The listing builds one solid part. Answer for the finished solid, in the listing's coordinates (mm). A direction names the side the tool comes from. Give positions to 0.01 mm unless a question says otherwise; leave off trailing zeros. Order: outer loops, then holes, each group sorted by start corner. A loop starts at its lowest first (then second) coordinate and runs counter-clockwise, first axis right, second up. Notation, with made-up numbers: (84.25, 22) - (118.25, 22) arc R13 cw to (118.25, 31) - close; hole circle Ø10 at (24, 9). An arc over 180 degrees is marked (long way). Answer as a JSON object with one key per item and string values. Group by question number.
Q1. The mould has two halves that part along Y. Classify faces 1 (the face through (12, 12, -2)), 2 (the face through (12, -1, 1)), 3 (the face through (24, 12, 1)), 4 (the face through (12, 25.5, 1)): released by +Y, released by -Y, zero draft, split by the parting line, or undercut.
Q2. Consider line 1 (Y direction, x = 9, z = 1.9); line 2 (X direction, y = 10.75, z = 1.45); line 3 (Z direction, x = 17, y = 14.5). Determine where each line is inside the solid, lowest interval first.
Q3. A cutting plane is placed at A-A, the plane z = 2.65. Give the vertices of the cut face in (x, y).
Q4. Given pin 1 (7 mm diameter, centred on x = 16, y = 13, fed in from +Z), flat-ended and moving along its own axis, determine where the tip first touches the part or whether it passes through.
Q5. A cutting plane is placed at B-B, the plane x = 2.5. Give the vertices of the cut face in (y, z).
Q6. A cutting plane is placed at C-C, the plane y = 20.75. Give the vertices of the cut face in (x, z).
Q7. For faces 5 (the face through (-0.6, 12.3, 3)), 6 (the face through (12, 12, 0)), determine the directions among +Z, -Z, +X, -X, +Y, -Y from which every point of the face is accessible in a straight line to the end or side of a thin tool.
from build123d import *

# Parameters (mm, degrees)
SKETCH_1_W      = 26
SKETCH_1_H      = 26.5
SKETCH_1_W_2    = 24
SKETCH_1_H_2    = 24.5
EXTRUDE_1_DEPTH = 3
SKETCH_2_W      = 26
SKETCH_2_H      = 26.5
EXTRUDE_2_DEPTH = 2


with BuildPart() as part:
    # 草图1 → 凸台-拉伸1 (new body)
    with BuildSketch(Plane.XY):
        with Locations((12, 12.25)):
            Rectangle(SKETCH_1_W, SKETCH_1_H)
        with Locations((12, 12.25)):
            Rectangle(SKETCH_1_W_2, SKETCH_1_H_2, mode=Mode.SUBTRACT)
    extrude(amount=EXTRUDE_1_DEPTH)

    # 草图2 → 凸台-拉伸2 (add)
    with BuildSketch(Plane(origin=(0, 0, 0), x_dir=(-1, 0, 0), z_dir=(0, 0, -1))):
        with Locations((-12, 12.25)):
            Rectangle(SKETCH_2_W, SKETCH_2_H)
    extrude(amount=EXTRUDE_2_DEPTH)


solid = part.part
Reply:
{
 "1": {"face 1": "zero draft", "face 2": "released by -Y", "face 3": "undercut", "face 4": "released by +Y"},
 "2": {"line 1": "y = -1 to 0, 24.5 to 25.5", "line 2": "x = -1 to 0, 24 to 25", "line 3": "z = -2 to 0"},
 "3": {"outline": "(-1, -1) - (25, -1) - (25, 25.5) - (-1, 25.5) - close; hole (0, 0) - (24, 0) - (24, 24.5) - (0, 24.5) - close"},
 "4": {"pin 1": "stops at z = 0"},
 "5": {"outline": "(-1, -2) - (25.5, -2) - (25.5, 3) - (24.5, 3) - (24.5, 0) - (0, 0) - (0, 3) - (-1, 3) - close"},
 "6": {"outline": "(-1, -2) - (25, -2) - (25, 3) - (24, 3) - (24, 0) - (0, 0) - (0, 3) - (-1, 3) - close"},
 "7": {"face 5": "+Z, +X, -X, +Y, -Y", "face 6": "+Z"}
}
